```python
from build123d import *

# Parameters (mm, degrees)
SKETCH1_R           = 30.25
SKETCH1_R_2         = 25.25
EXTRUDE_THIN1_DEPTH = 2
SKETCH2_R           = 1.65
CUT_EXTRUDE3_DEPTH  = 10
BOSS_EXTRUDE1_DEPTH = 2


with BuildPart() as part:
    # Sketch1 → Extrude-Thin1 (new body)
    with BuildSketch(Plane(origin=(0, 0, 0), x_dir=(1, 0, 0), z_dir=(0, 1, 0))):
        Circle(SKETCH1_R)
        Circle(SKETCH1_R_2, mode=Mode.SUBTRACT)
    extrude(amount=-EXTRUDE_THIN1_DEPTH)

    # Sketch2 → Cut-Extrude3 (cut)
    with BuildSketch(Plane(origin=(0, 0, 0), x_dir=(1, 0, 0), z_dir=(0, 1, 0))):
        with Locations((0, 27.5)):
            Circle(SKETCH2_R)
        with Locations((23.815698604, -13.75)):
            Circle(SKETCH2_R)
        with Locations((-23.815698604, -13.75)):
            Circle(SKETCH2_R)
    extrude(amount=-CUT_EXTRUDE3_DEPTH, mode=Mode.SUBTRACT)

    # Sketch5 → Boss-Extrude1 (add)
    with BuildSketch(Plane.XZ.offset(2)):
        with BuildLine():
            Line((0, 55.25), (0, 30.25))
            ThreePointArc((0, 30.25), (3.686547638, 30.024521087), (7.318137342, 29.35144572))
            Line((7.318137342, 29.35144572), (13.366184732, 53.608838877))
            ThreePointArc((13.366184732, 53.608838877), (6.733281223, 54.838174878), (0, 55.25))
        make_face()
        with BuildLine():
            Line((35.514015435, 42.323955482), (19.444325193, 23.172844404))
            ThreePointArc((19.444325193, 23.172844404), (22.123449474, 20.630450392), (24.47276408, 17.780503882))
            Line((24.47276408, 17.780503882), (44.698188939, 32.475135189))
            ThreePointArc((44.698188939, 32.475135189), (40.407292014, 37.680409393), (35.514015435, 42.323955482))
        make_face()
        with BuildLine():
            Line((54.410628354, 9.594061816), (29.790434529, 5.252857374))
            ThreePointArc((29.790434529, 5.252857374), (30.208543426, 1.583162676), (30.17631252, -2.110133331))
            Line((30.17631252, -2.110133331), (55.115413777, -3.854045174))
            ThreePointArc((55.115413777, -3.854045174), (55.174281795, 2.891561582), (54.410628354, 9.594061816))
        make_face()
        with BuildLine():
            Line((47.847903559, -27.625), (26.197268464, -15.125))
            ThreePointArc((26.197268464, -15.125), (24.158724179, -18.20490445), (21.76002896, -21.013415706))
            Line((21.76002896, -21.013415706), (39.743523969, -38.379874968))
            ThreePointArc((39.743523969, -38.379874968), (44.12461193, -33.250280029), (47.847903559, -27.625))
        make_face()
        with BuildLine():
            Line((18.896612919, -51.918017298), (10.346109336, -28.425701779))
            ThreePointArc((10.346109336, -28.425701779), (6.804769394, -29.47469446), (3.161986014, -30.084287335))
            Line((3.161986014, -30.084287335), (5.775197596, -54.947334719))
            ThreePointArc((5.775197596, -54.947334719), (12.428545752, -53.833946079), (18.896612919, -51.918017298))
        make_face()
        with BuildLine():
            Line((-18.896612919, -51.918017298), (-10.346109336, -28.425701779))
            ThreePointArc((-10.346109336, -28.425701779), (-13.733212617, -26.952947357), (-16.91558533, -25.07838657))
            Line((-16.91558533, -25.07838657), (-30.895407917, -45.804325884))
            ThreePointArc((-30.895407917, -45.804325884), (-25.082975111, -49.228110461), (-18.896612919, -51.918017298))
        make_face()
        with BuildLine():
            Line((-47.847903559, -27.625), (-26.197268464, -15.125))
            ThreePointArc((-26.197268464, -15.125), (-27.845271817, -11.819616637), (-29.078166302, -8.338030013))
            Line((-29.078166302, -8.338030013), (-53.109708701, -15.228963909))
            ThreePointArc((-53.109708701, -15.228963909), (-50.857893153, -21.587894849), (-47.847903559, -27.625))
        make_face()
        with BuildLine():
            Line((-54.410628354, 9.594061816), (-29.790434529, 5.252857374))
            ThreePointArc((-29.790434529, 5.252857374), (-28.928218868, 8.844244068), (-27.634750094, 12.303783453))
            Line((-27.634750094, 12.303783453), (-50.473386535, 22.47219953))
            ThreePointArc((-50.473386535, 22.47219953), (-52.835837767, 16.153536686), (-54.410628354, 9.594061816))
        make_face()
        with BuildLine():
            Line((-35.514015435, 42.323955482), (-19.444325193, 23.172844404))
            ThreePointArc((-19.444325193, 23.172844404), (-16.475330809, 25.36978468), (-13.26072719, 27.188519901))
            Line((-13.26072719, 27.188519901), (-24.22000586, 49.658371058))
            ThreePointArc((-24.22000586, 49.658371058), (-30.091306685, 46.336548879), (-35.514015435, 42.323955482))
        make_face()
    extrude(amount=-BOSS_EXTRUDE1_DEPTH)


solid = part.part
```
Here's how the part is built. I have some questions about the finished solid (model axes, mm). A direction names the side the tool comes from. Give positions to 0.01 mm unless a question says otherwise; leave off trailing zeros. Write each loop counter-clockwise with the first axis right and the second up, starting at its lowest first coordinate (ties: lowest second). Pieces come first, ordered by that corner, then holes. Notation, with made-up numbers: M 24.5,14.5 L 53.5,14.5 A29 ccw 53.5,41.5 Z; hole C 8,-2.5 d7. An arc over 180 degrees is marked long. Put each result on its own line as item: value. Start each with the question number.
Item 1: Thinking about a two-plate mould opening in Z: for faces 1 (the flat face through (34.44, -1.01, 25.02)), 2 (the cylindrical face through (-50.895, -1.014, -21.501)), 3 (the cylindrical face through (-6.898, -0.986, 29.453)), which applies, +Z half, -Z half, draft (parallel to the pull), parting line (faces both ways), or undercut?
Item 2: If we section it at D-D, the plane x = 43: Write out the boundary of the cut face in (y, z), then the cut area to 3 significant figures.
Item 3: If we section it at B-B, the plane z = -34: Write out the boundary of the cut face in (x, y).
Item 4: If we section it at C-C, the plane z = 13.75: Write out the boundary of the cut face in (x, y), then the cut area to 3 significant figures.
Item 5: On a 3-axis mill with a long thin cutter (end or side, diameter ignored), from which of +Z, -Z, +X, -X, +Y, -Y can I reach the whole of each face in a straight line? I mean faces 4 (the cylindrical face through (16.556, -0.986, -25.317)), 5 (the flat face through (4.45, -1.01, -42.34)), 6 (the flat face through (-42.273, -1.014, 7.454)), 7 (the flat face through (27.59, -1.01, 32.88)), 8 (the cylindrical face through (-52.81, -1.01, 16.24)). Say none if no direction works.
Item 6: Will these pins go through, and if not, where does the flat tip stop? pin 1 (1 mm diameter, centred on y = -0.5, z = 39, fed in from -X); pin 2 (1 mm diameter, centred on x = -25, y = -0.5, fed in from +Z).
Item 7: If we section it at A-A, the plane z = 0: Write out the boundary of the cut face in (x, y), then the cut area to 3 significant figures.
Item 8: I need wall thicknesses on L1, parallel to Z at x = 40.5, y = -0.2; L2, parallel to X at y = -1, z = -27.5; L3, parallel to Z at x = -22, y = -1.8. Which ranges of each line are inside material? Lowest first, please. Write a range as from..to.
Values:
1. face 1: undercut
1. face 2: -Z half
1. face 3: +Z half
2. outline: M -2,-34.69 L 0,-34.69 L 0,-24.83 L -2,-24.83 Z; M -2,-3.01 L 0,-3.01 L 0,7.58 L -2,7.58 Z; M -2,31.24 L 0,31.24 L 0,34.69 L -2,34.69 Z
2. area: 47.8 mm²
3. outline: M -22.93,-2 L -12.37,-2 L -12.37,0 L -22.93,0 Z; M 3.57,-2 L 12.37,-2 L 12.37,0 L 3.57,0 Z; M 35.21,-2 L 43.55,-2 L 43.55,0 L 35.21,0 Z
4. outline: M -53.51,-2 L -30.88,-2 L -30.88,0 L -53.51,0 Z; M -26.94,-2 L -25.47,-2 L -25.47,0 L -26.94,0 Z; M -22.17,-2 L -21.18,-2 L -21.18,0 L -22.17,0 Z; M 21.18,-2 L 22.17,-2 L 22.17,0 L 21.18,0 Z; M 25.47,-2 L 26.94,-2 L 26.94,0 L 25.47,0 Z
4. area: 55.1 mm²
5. face 4: +Y, -Y
5. face 5: -Z, +Y, -Y
5. face 6: -X, +Y, -Y
5. face 7: +Z, +Y, -Y
5. face 8: +Z, -X, +Y, -Y
6. pin 1: x = -33.14
6. pin 2: z = 49.52
7. outline: M -30.25,-2 L -25.25,-2 L -25.25,0 L -30.25,0 Z; M 25.25,-2 L 55.25,-2 L 55.25,0 L 25.25,0 Z
7. area: 70.0 mm²
8. L1: -37.58..-23.38, -2.83..7.14, 29.42..37.58
8. L2: -47.92..-47.63, -18.55..-1.65, 1.65..12.6, 28.48..47.63
8. L3: -50.68..-32.62, -20.76..-12.39, 12.39..20.76, 26.22..45.11
